Source: CAD feature listing. Evaluate the final solid. Frame: model axes, mm. A direction names the side the tool comes from. Round coordinates to 2 decimals unless told otherwise and drop trailing zeros. Loops run counter-clockwise (first coordinate to the right, second up) from the corner with the lowest first, then second, coordinate; pieces in that order, holes last. Notation, with made-up numbers: (53.5, 34) - (80.5, 34) arc R30 cw to (80.5, 56) - close; hole circle Ø5 at (-34, 44). An arc over 180 degrees is marked (long way). One line per question, with ' | ' between items.
from build123d import *

# Parameters (mm, degrees)
F0_R     = 12.7
F0_R_2   = 10.16
F0_R_3   = 7.9375
F0_R_4   = 3.3782
F1_DEPTH = 8.89
F2_DEPTH = 12.192
F3_DEPTH = 25.4
F4_DEPTH = 2.54
F5_SIZE  = 0.762
F7_DEPTH = 7.62


with BuildPart() as f1:
    # F0 (on Top) → F1 (new body)
    with BuildSketch(Plane.XY):
        Circle(F0_R)
        Circle(F0_R_2, mode=Mode.SUBTRACT)
        Circle(F0_R_2)
        Circle(F0_R_3, mode=Mode.SUBTRACT)
        Circle(F0_R_3)
        with Locations((0, 0.150276348)):
            Circle(F0_R_4, mode=Mode.SUBTRACT)
        with Locations((0, 0.150276348)):
            Circle(F0_R_4)
    extrude(amount=F1_DEPTH)

    # F0 (on Top) → F2 (join)
    with BuildSketch(Plane.XY):
        Circle(F0_R_3)
        with Locations((0, 0.150276348)):
            Circle(F0_R_4, mode=Mode.SUBTRACT)
        with Locations((0, 0.150276348)):
            Circle(F0_R_4)
    extrude(amount=F2_DEPTH)

    # F0 (on Top) → F3 (cut)
    with BuildSketch(Plane.XY):
        with Locations((0, 0.150276348)):
            Circle(F0_R_4)
    extrude(amount=F3_DEPTH, mode=Mode.SUBTRACT)

    # F0 (on Top) → F4 (cut)
    with BuildSketch(Plane.XY):
        Circle(F0_R_2)
        Circle(F0_R_3, mode=Mode.SUBTRACT)
        Circle(F0_R_3)
        with Locations((0, 0.150276348)):
            Circle(F0_R_4, mode=Mode.SUBTRACT)
    extrude(amount=F4_DEPTH, mode=Mode.SUBTRACT)

    # F5
    f5_edges = [f1.edges().sort_by_distance(p)[0] for p in [
        (-7.9375, 0, 12.192),
    ]]
    chamfer(f5_edges, length=F5_SIZE)

    # F6 (on Top) → F7 (cut)
    with BuildSketch(Plane.XY):
        Polygon((3.1749068653, 5.4991), (-3.1749068653, 5.4991), (-6.3498137306, 0), (-3.1749068653, -5.4991), (3.1749068653, -5.4991), (6.3498137306, 0), align=None)
    extrude(amount=F7_DEPTH, mode=Mode.SUBTRACT)


solid = f1.part
1. Contact query for flat-ended pins moving along their axis: P1, Ø3, axis at y = 8.5, z = 8, coming from the -X side; P2, Ø6, axis at y = -5, z = 9.5, coming from the +X side; P3, Ø5.5, axis at x = 1, y = 0.5, coming from the -Z side; P4, Ø3, axis at x = -10, z = 11, coming from the -Y side. Output: stop coordinate, or through.
Worked out:
P1: stops at x = -10.6 | P2: stops at x = 12.53 | P3: stops at z = 7.62 | P4: passes through
2. Section query B-B, the plane z = 10.75. Return loops of the section in (x, y) (1 decimal), plus the area to 3 significant figures.
Worked out:
outline: circle Ø15.9 at (0, 0); hole circle Ø6.8 at (0, 0.2) | area: 162 mm2
3. Section query C-C, the plane y = 11. Return loops of the section in (x, z).
Worked out:
outline: (-6.35, 0) - (6.35, 0) - (6.35, 8.89) - (-6.35, 8.89) - close
4. Mould query, pull axis Y, two halves, no side actions, for faces 4 (the cylindrical face through (-3.375, 0.299, 9.874)), 5 (the flat face through (1.5, -3.1, 12.192)), 6 (the cylindrical face through (-2.75, -12.4, 4.38)). Classes: released by +Y, released by -Y, zero draft, split by the parting line, or undercut.
Worked out:
face 4: undercut | face 5: zero draft | face 6: split by the parting line
5. Access query for faces 1 (the flat face through (-6, 9, 0)), 2 (the cylindrical face through (-1.323, 10.074, 1.252)), 3 (the flat face through (-0.2, -8.3, 8.89)). Directions: +Z, -Z, +X, -X, +Y, -Y. A direction counts if a zero-diameter tool reaches every point of the face in a straight line with its end or side. Return the directions, or none.
Worked out:
face 1: -Z, +X, -X, +Y, -Y | face 2: -Z | face 3: +Z
6. Section query A-A, the plane x = 0. Return loops of the section in (y, z), plus the area to 3 significant figures.
Worked out:
outline: (-12.7, 0) - (-10.16, 0) - (-10.16, 2.54) - (-5.5, 2.54) - (-5.5, 7.62) - (-3.23, 7.62) - (-3.23, 12.19) - (-7.18, 12.19) - (-7.94, 11.43) - (-7.94, 8.89) - (-12.7, 8.89) - close; (3.53, 7.62) - (5.5, 7.62) - (5.5, 2.54) - (10.16, 2.54) - (10.16, 0) - (12.7, 0) - (12.7, 8.89) - (7.94, 8.89) - (7.94, 11.43) - (7.18, 12.19) - (3.53, 12.19) - close | area: 139 mm2
7. Material intervals for probe 1 along Y at (x, z) = (0, 10.35); probe 2 along Y at (x, z) = (0.25, 6); probe 3 along Z at (x, y) = (2, 11.25), sorted ascending.
Worked out:
probe 1: y = -7.94 to -3.23, 3.53 to 7.94 | probe 2: y = -12.7 to -5.5, 5.5 to 12.7 | probe 3: z = 0 to 8.89
